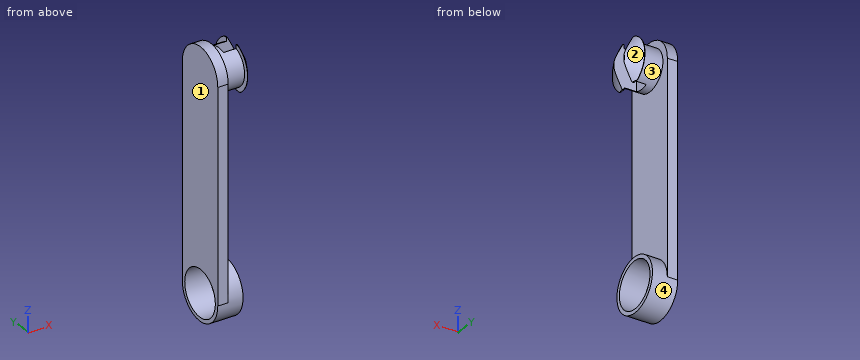
from build123d import *

# Parameters (mm, degrees)
F0_R      = 1.55
F1_DEPTH  = 0.7
F2_R      = 1.35
F3_DEPTH  = 1.4
F4_R      = 1.65
F5_DEPTH  = 0.65
F6_SIZE2  = 0.6350852961
F6_SIZE   = 1.1
F8_DEPTH  = 1.5
F9_R      = 1.8
F9_R_2    = 1.55
F10_DEPTH = 1


with BuildPart() as f1:
    # F0 (on Right) → F1 (new body)
    with BuildSketch(Plane.YZ):
        with BuildLine():
            Line((1.8, -7), (1.8, 7))
            ThreePointArc((1.8, 7), (0, 8.8), (-1.8, 7))
            Line((-1.8, 7), (-1.8, -7))
            ThreePointArc((-1.8, -7), (0, -8.8), (1.8, -7))
        make_face()
        with Locations((0, -7)):
            Circle(F0_R, mode=Mode.SUBTRACT)
    extrude(amount=F1_DEPTH)

    # F2 (on face) → F3 (join)
    with BuildSketch(Plane.YZ.offset(0.7)):
        with Locations((0, 7)):
            Circle(F2_R)
    extrude(amount=F3_DEPTH)

    # F4 (on face) → F5 (join)
    with BuildSketch(Plane.YZ.offset(2.1)):
        with Locations((0, 7)):
            Circle(F4_R)
    extrude(amount=F5_DEPTH)

    # F6
    f6_edges = [f1.edges().sort_by_distance(p)[0] for p in [
        (2.75, -1.65, 7),
    ]]
    f6_side = f1.faces().sort_by_distance((2.75, 0, 7))[0]
    chamfer(f6_edges, length=F6_SIZE, length2=F6_SIZE2, reference=f6_side)

    # F7 (on face) → F8 (cut)
    with BuildSketch(Plane.YZ.offset(2.75)):
        with BuildLine():
            Line((0.5, 8.8), (-0.5, 8.8))
            Line((-0.5, 8.8), (-1, 8.8))
            Line((-1, 8.8), (-1, 8.5))
            Line((-1, 8.5), (-0.5, 8.5))
            Line((-0.5, 8.5), (-0.5, 7.2291287847))
            ThreePointArc((-0.5, 7.2291287847), (0, 7.55), (0.5, 7.2291287847))
            Line((0.5, 7.2291287847), (0.5, 8.5))
            Line((0.5, 8.5), (1, 8.5))
            Line((1, 8.5), (1, 8.8))
            Line((1, 8.8), (0.5, 8.8))
        make_face()
        with BuildLine():
            ThreePointArc((0.5, 7.2291287847), (0, 7.55), (-0.5, 7.2291287847))
            Line((-0.5, 7.2291287847), (-0.5, 6.7708712153))
            ThreePointArc((-0.5, 6.7708712153), (0, 6.45), (0.5, 6.7708712153))
            Line((0.5, 6.7708712153), (0.5, 7.2291287847))
        make_face()
        with BuildLine():
            ThreePointArc((0.5, 6.7708712153), (0, 6.45), (-0.5, 6.7708712153))
            Line((-0.5, 6.7708712153), (-0.5, 5.6))
            Line((-0.5, 5.6), (-1, 5.6))
            Line((-1, 5.6), (-1, 5.3))
            Line((-1, 5.3), (-0.5, 5.3))
            Line((-0.5, 5.3), (0.5, 5.3))
            Line((0.5, 5.3), (1, 5.3))
            Line((1, 5.3), (1, 5.6))
            Line((1, 5.6), (0.5, 5.6))
            Line((0.5, 5.6), (0.5, 6.7708712153))
        make_face()
    extrude(amount=-F8_DEPTH, mode=Mode.SUBTRACT)

    # F9 (on face) → F10 (join)
    with BuildSketch(Plane.YZ.offset(0.7)):
        with Locations((0, -7)):
            Circle(F9_R)
        with Locations((0, -7)):
            Circle(F9_R_2, mode=Mode.SUBTRACT)
    extrude(amount=F10_DEPTH)


solid = f1.part
Geometry check sheet. Reference: the model listing, model coordinates, mm. Face numbers are marked on the shaded views. Give positions to 0.01 mm unless a question says otherwise; leave off trailing zeros. Write each loop counter-clockwise with the first axis right and the second up, starting at its lowest first coordinate (ties: lowest second). Pieces come first, ordered by that corner, then holes.
1) Cross-section at A-A (y = 0). Record the boundary of the cut face in (x, z), plus the area to 3 significant figures.
Values follow:
outline: (0, -8.8) - (1.7, -8.8) - (1.7, -8.55) - (0, -8.55) - close; (0, -5.45) - (1.7, -5.45) - (1.7, -5.2) - (0.7, -5.2) - (0.7, 5.65) - (1.25, 5.65) - (1.25, 8.35) - (0.7, 8.35) - (0.7, 8.8) - (0, 8.8) - close
area: 12.1 mm2
2) Go/stop test with flat-tipped pins: pin 1 Ø1.2 at (x, z) = (2, 6.5) entering from -Y; pin 2 Ø1 at (x, y) = (1.5, -1) entering from -Z; pin 3 Ø1.8 at (y, z) = (0, -6.5) entering from +X; pin 4 Ø0.9 at (y, z) = (-1, 6.5) entering from -X. Record where each tip stops, or that it passes through.
Values follow:
pin 1: stops at y = -1.65
pin 2: stops at z = -8.73
pin 3: passes through
pin 4: stops at x = 0
3) Cross-section at B-B (x = 0.9). Record the boundary of the cut face in (y, z).
Values follow:
outline: circle Ø3.6 at (0, -7); circle Ø2.7 at (0, 7); hole circle Ø3.1 at (0, -7)
4) Cross-section at C-C (z = -4.5). Record the boundary of the cut face in (x, y), plus the area to 3 significant figures.
Values follow:
outline: (0, -1.8) - (0.7, -1.8) - (0.7, 1.8) - (0, 1.8) - close
area: 2.52 mm2
5) Release check for a two-part mould opening along X. For the marked faces 1, 2, 3 and 4 record: released by +X, released by -X, zero draft, split by the parting line, or undercut.
Values follow:
face 1: released by -X
face 2: released by +X
face 3: undercut
face 4: zero draft
6) Thickness scan on line 1 (Z direction, x = 1, y = 0); line 2 (Z direction, x = 1.5, y = -1.1); line 3 (Z direction, x = 0.5, y = 0). Record the ranges inside material, lowest first.
Values follow:
line 1: z = -8.8 to -8.55, -5.45 to -5.2, 5.65 to 8.35
line 2: z = -8.42 to -8.09, -5.91 to -5.58, 6.22 to 7.78
line 3: z = -8.8 to -8.55, -5.45 to 8.8
7) Cross-section at D-D (x = 2.5). Record the boundary of the cut face in (y, z).
Values follow:
outline: (-0.5, 6.15) - (-0.5, 7.85) arc R0.98 ccw to start; (0.5, 6.15) arc R0.98 ccw to (0.5, 7.85) - close
